from build123d import *

# Parameters (mm, degrees)
SKETCH1_W           = 48
SKETCH1_H           = 53
SKETCH1_R           = 1.9304
BOSS_EXTRUDE1_DEPTH = 10
SKETCH2_W           = 48
SKETCH2_H           = 5.616325
BOSS_EXTRUDE2_DEPTH = 33.1917878
SKETCH4_W           = 4
SKETCH4_H           = 10
BOSS_EXTRUDE4_DEPTH = 40
SKETCH5_W           = 48
SKETCH5_H           = 10.8609375
BOSS_EXTRUDE5_DEPTH = 23.1917878
SKETCH6_W           = 48
SKETCH6_H           = 5
BOSS_EXTRUDE6_DEPTH = 42.3
CUT_EXTRUDE1_REACH  = 78.862
SKETCH8_R           = 11.5
SKETCH9_R           = 1.9304
CUT_EXTRUDE2_DEPTH  = 88.252507127
CUT_EXTRUDE3_REACH  = 89.253
SKETCH10_W          = 3.15468
SKETCH10_H          = 6.8326
BOSS_EXTRUDE7_START = 8
SKETCH11_W          = 48
SKETCH11_H          = 42.3
SKETCH11_R          = 11.5
BOSS_EXTRUDE7_DEPTH = 8
SKETCH12_W          = 48
SKETCH12_H          = 42.3
BOSS_EXTRUDE8_DEPTH = 8
FILLET1_R           = 11
BOSS_EXTRUDE9_DEPTH = 3
CUT_EXTRUDE4_DEPTH  = 6


with BuildPart() as part:
    # Sketch1 → Boss-Extrude1 (new body)
    with BuildSketch(Plane.XY):
        with Locations((24, 26.5)):
            Rectangle(SKETCH1_W, SKETCH1_H)
        with Locations((8.975, 38)):
            Circle(SKETCH1_R, mode=Mode.SUBTRACT)
        with Locations((38.975, 38)):
            Circle(SKETCH1_R, mode=Mode.SUBTRACT)
    extrude(amount=BOSS_EXTRUDE1_DEPTH)

    # Sketch2 → Boss-Extrude2 (add)
    with BuildSketch(Plane(origin=(0, 0, 0), x_dir=(-1, 0, 0), z_dir=(0, 0, -1))):
        with Locations((-24, -2.8081625)):
            Rectangle(SKETCH2_W, SKETCH2_H)
    extrude(amount=-BOSS_EXTRUDE2_DEPTH)

    # Sketch4 → Boss-Extrude4 (add)
    with BuildSketch(Plane.XY.offset(10)):
        with Locations((2, 48)):
            Rectangle(SKETCH4_W, SKETCH4_H)
        with Locations((46, 48)):
            Rectangle(SKETCH4_W, SKETCH4_H)
    extrude(amount=BOSS_EXTRUDE4_DEPTH)

    # Sketch5 → Boss-Extrude5 (add)
    with BuildSketch(Plane.XY.offset(10)):
        with Locations((24, 5.43046875)):
            Rectangle(SKETCH5_W, SKETCH5_H)
    extrude(amount=BOSS_EXTRUDE5_DEPTH)

    # Sketch6 → Boss-Extrude6 (add)
    with BuildSketch(Plane.XZ.offset(5.616325)):
        with Locations((24, 30.6917878)):
            Rectangle(SKETCH6_W, SKETCH6_H)
    extrude(amount=BOSS_EXTRUDE6_DEPTH)

    # Sketch8 → Cut-Extrude1 (cut, up to next)
    with BuildSketch(Plane(origin=(0, 0, 28.1917878), x_dir=(-1, 0, 0), z_dir=(0, 0, -1)), mode=Mode.PRIVATE) as cut_extrude1_sk1:
        with Locations((-24, -26.616325)):
            Circle(SKETCH8_R)
    cut_extrude1_tool1 = extrude(cut_extrude1_sk1.sketch, amount=-CUT_EXTRUDE1_REACH, mode=Mode.PRIVATE) & part.part
    add(cut_extrude1_tool1.solids().sort_by_distance((24, -26.616325, 28.191788))[0], mode=Mode.SUBTRACT)

    # Sketch9 → Cut-Extrude2 (cut, through all)
    with BuildSketch(Plane(origin=(48, 0, 0), x_dir=(0, 0, -1), z_dir=(1, 0, 0))):
        with Locations((-17, 48)):
            Circle(SKETCH9_R)
    extrude(amount=-CUT_EXTRUDE2_DEPTH, mode=Mode.SUBTRACT)

    # Sketch10 → Cut-Extrude3 (cut, up to next)
    with BuildSketch(Plane(origin=(0, 0, 0), x_dir=(-1, 0, 0), z_dir=(0, 0, -1)), mode=Mode.PRIVATE) as cut_extrude3_sk1:
        with Locations((-35.42266, 48)):
            Rectangle(SKETCH10_W, SKETCH10_H)
    cut_extrude3_tool1 = extrude(cut_extrude3_sk1.sketch, amount=-CUT_EXTRUDE3_REACH, mode=Mode.PRIVATE) & part.part
    # Sketch10 → Cut-Extrude3 (cut, up to next)
    with BuildSketch(Plane(origin=(0, 0, 0), x_dir=(-1, 0, 0), z_dir=(0, 0, -1)), mode=Mode.PRIVATE) as cut_extrude3_sk2:
        with Locations((-12.57734, 48)):
            Rectangle(SKETCH10_W, SKETCH10_H)
    cut_extrude3_tool2 = extrude(cut_extrude3_sk2.sketch, amount=-CUT_EXTRUDE3_REACH, mode=Mode.PRIVATE) & part.part
    add(cut_extrude3_tool1.solids().sort_by_distance((35.42266, 48, 0))[0], mode=Mode.SUBTRACT)
    add(cut_extrude3_tool2.solids().sort_by_distance((12.57734, 48, 0))[0], mode=Mode.SUBTRACT)

    # Sketch11 → Boss-Extrude7 (add)
    with BuildSketch(Plane(origin=(0, 0, 28.1917878), x_dir=(-1, 0, 0), z_dir=(0, 0, -1)).offset(BOSS_EXTRUDE7_START)):
        with Locations((-24, -26.766325)):
            Rectangle(SKETCH11_W, SKETCH11_H)
        with Locations((-24, -26.616325)):
            Circle(SKETCH11_R, mode=Mode.SUBTRACT)
    extrude(amount=-BOSS_EXTRUDE7_DEPTH)

    # Sketch12 → Boss-Extrude8 (add)
    with BuildSketch(Plane(origin=(0, 0, 20.1917878), x_dir=(-1, 0, 0), z_dir=(0, 0, -1))):
        with Locations((-24, -26.766325)):
            Rectangle(SKETCH12_W, SKETCH12_H)
    extrude(amount=BOSS_EXTRUDE8_DEPTH)

    # Fillet1
    fillet1_edges = [part.edges().sort_by_distance(p)[0] for p in [
        (24, -5.616325, 0),
    ]]
    fillet(fillet1_edges, radius=FILLET1_R)

    # Sketch13 → Boss-Extrude9 (add)
    with BuildSketch(Plane(origin=(0, 53, 0), x_dir=(1, 0, 0), z_dir=(0, 1, 0))):
        Polygon((0, 0), (0, -50), (4, -50), (4, -10), (44, -10), (44, -50), (48, -50), (48, 0), align=None)
    extrude(amount=BOSS_EXTRUDE9_DEPTH)

    # Sketch14 → Cut-Extrude4 (cut)
    with BuildSketch(Plane.XY.offset(10)):
        Polygon((8.975, 41.9594682), (5.545999953, 39.9797341), (5.545999953, 36.0202659), (8.975, 34.0405318), (12.404000047, 36.0202659), (12.404000047, 39.9797341), align=None)
        Polygon((38.975, 41.9594682), (35.545999953, 39.9797341), (35.545999953, 36.0202659), (38.975, 34.0405318), (42.404000047, 36.0202659), (42.404000047, 39.9797341), align=None)
    extrude(amount=-CUT_EXTRUDE4_DEPTH, mode=Mode.SUBTRACT)


solid = part.part
Model file for the job. Use its own axes, mm. A direction names the side the tool comes from. Give positions to 0.01 mm unless a question says otherwise; leave off trailing zeros. Loops run counter-clockwise (first coordinate to the right, second up) from the corner with the lowest first, then second, coordinate; pieces in that order, holes last. Notation, with made-up numbers: (-15.5, -10.5) - (7.5, -10.5) arc R21 ccw to (7.5, 11.5) - close; hole circle Ø5 at (-16.5, 26). An arc over 180 degrees is marked (long way). Use one line per item in the form item = value.
(1) Drill centre lines: L1, parallel to Y at x = 45.45, z = 17; L2, parallel to X at y = 38, z = 1; L3, parallel to X at y = 39, z = 6. Where is each one in solid material? Low to high.
Determined:
L1 = -47.92 to 10.86, 43 to 46.07, 49.93 to 56
L2 = 0 to 7.04, 10.91 to 37.04, 40.91 to 48
L3 = 0 to 5.55, 12.4 to 35.55, 42.4 to 48
(2) Cut at B-B (z = 17). Give the cut face in (x, y).
Determined:
outline = (0, -47.92) - (48, -47.92) - (48, 10.86) - (0, 10.86) - close; (0, 43) - (4, 43) - (4, 46.07) - (0, 46.07) - close; (0, 49.93) - (4, 49.93) - (4, 56) - (0, 56) - close; (44, 43) - (48, 43) - (48, 46.07) - (44, 46.07) - close; (44, 49.93) - (48, 49.93) - (48, 56) - (44, 56) - close
(3) Cut at C-C (z = 40). Give the cut face in (x, y).
Determined:
outline = (0, 43) - (4, 43) - (4, 56) - (0, 56) - close; (44, 43) - (48, 43) - (48, 56) - (44, 56) - close
(4) Pull direction Y, two halves, no side cores. Call faces 1 (the face through (0, 3, 19)), 2 (the face through (24, -47.916, 23)), 3 (the face through (8.724, 39.914, 1.972)): pulls with the +Y half, pulls with the -Y half, needs draft (parallel to the pull), parting line crosses it, or undercut.
Determined:
face_1 = needs draft
face_2 = pulls with the -Y half
face_3 = undercut
(5) 3-axis set-ups, long thin cutter, end or side, ignore diameter. For faces 4 (the face through (33.845, 48, 5)), 5 (the face through (24, 10.861, 21)), 6 (the face through (48, 3, 20)), 7 (the face through (23.66, -2.31, 3.14)), 8 (the face through (5.546, 38, 7)): which of +Z, -Z, +X, -X, +Y, -Y reach the whole face in a straight line?
Determined:
face_4 = +Z, -Z
face_5 = +Z, +X, -X
face_6 = +Z, -Z, +X, +Y, -Y
face_7 = -Z, +X, -X, -Y
face_8 = +Z
(6) Drop flat-ended pins along their axis: P1, Ø6, axis at x = 17.5, z = 26.5, coming from the +Y side; P2, Ø7.5, axis at x = 38.5, y = 36.5, coming from the +Z side; P3, Ø0.9, axis at x = 13, z = 5.5, coming from the -Y side. Give the stop position or say it passes through.
Determined:
P1 = 10.86
P2 = 10
P3 = -4.39
(7) Cut at D-D (x = 24). Give the cut face in (y, z), then the cut area to 3 significant figures.
Determined:
outline = (-47.92, 12.19) - (-5.62, 12.19) - (-5.62, 11) arc R11 ccw to (5.38, 0) - (56, 0) - (56, 10) - (10.86, 10) - (10.86, 33.19) - (-15.12, 33.19) - (-15.12, 20.19) - (-38.12, 20.19) - (-38.12, 33.19) - (-47.92, 33.19) - close
area = 1,560 mm^2
(8) Cut at A-A (y = 48). Give the cut face in (x, z), then the cut area to 3 significant figures.
Determined:
outline = (0, 0) - (11, 0) - (11, 10) - (4, 10) - (4, 15.07) - (0, 15.07) - close; (0, 18.93) - (4, 18.93) - (4, 50) - (0, 50) - close; (14.15, 0) - (33.85, 0) - (33.85, 10) - (14.15, 10) - close; (37, 0) - (48, 0) - (48, 15.07) - (44, 15.07) - (44, 10) - (37, 10) - close; (44, 18.93) - (48, 18.93) - (48, 50) - (44, 50) - close
area = 706 mm^2
